Solid Edge part; units mm, degrees
sketch "Sketch1" plane through (0, 0, 0) normal (0, -1, 0) x (1, 0, 0)
  line L0 (-402.4784, 77.6999) -> (-342.4784, 77.6999)
  line L1 (-342.4784, 77.6999) -> (-342.4784, 477.6999)
  line L2 (-342.4784, 477.6999) -> (-402.4784, 477.6999)
  line L3 (-402.4784, 477.6999) -> (-402.4784, 77.6999)
  line L4 (-412.4784, 57.6999) -> (-332.4784, 57.6999)
  line L5 (-332.4784, 57.6999) -> (-332.4784, 587.6999)
  line L6 (-332.4784, 587.6999) -> (-412.4784, 587.6999)
  line L7 (-412.4784, 587.6999) -> (-412.4784, 57.6999)
  dimension "D1" = 402.4784
  dimension "D2" = 342.4784
  dimension "D3" = 332.4784
  dimension "D4" = 412.4784
extrude "Protrusion1" add sketch "Sketch1" against normal blind 50
sketch "Sketch2" plane through (-372.4784, 25, 77.6999) normal (0, 0, 1) x (1, 0, 0)
  circle A0 centre (0, 0) radius 10
extrude "Protrusion2" add sketch "Sketch2" along normal up to surface (400 mm away)
sketch "Sketch3" plane through (-372.4784, 50, 247.6999) normal (0, 1, 0) x (0, 0, 1)
  line L0 (290, -40) -> (340, -40)
  line L1 (340, -40) -> (340, 40)
  line L2 (340, 40) -> (290, 40)
  line L3 (290, 40) -> (290, -40)
  dimension "D1" = 290
  dimension "D2" = 340
extrude "ExtrudedProtrusion_3" add sketch "Sketch3" along normal blind 270
sketch "Sketch4" plane through (-372.4784, 310, 587.6999) normal (0, 0, 1) x (0, 1, 0)
  circle A0 centre (10, 0) radius 50
extrude "Cutout1" cut sketch "Sketch4" against normal through all
Design review of the part built by this model. Coordinates are the model's own, in mm. A direction names the side the tool comes from. Coordinates: 2 decimals unless noted, no trailing zeros. Order: outer loops, then holes, each group sorted by start corner. A loop starts at its lowest first (then second) coordinate and runs counter-clockwise, first axis right, second up. Notation, with made-up numbers: M -34.5,82.5 L -2.5,82.5 A32 ccw -2.5,112.5 Z; hole C -30,5.25 d5. An arc over 180 degrees is marked long. Answer as a JSON object with one key per item and string values. Group by question number.
1) Add section C-C, the plane x = -357.5. Write out the cut boundary in (y, z), then the cut area to 3 significant figures.
2) Tool access review of faces 1 (the flat face through (-372, 14, 477.7)), 2 (the flat face through (-342.478, 25, 275)), 3 (the flat face through (-340, 50, 334)): name each direction out of +Z, -Z, +X, -X, +Y, -Y from which nothing blocks a thin tool from reaching the whole face with its end or side.
3) Add section D-D, the plane y = 188.5. Write out the cut boundary in (x, z).
4) Wall thickness on L1, parallel to Z at x = -348, y = 122.5; L2, parallel to X at y = 32.5, z = 307; L3, parallel to Y at x = -403, z = 479: over which ranges is each line inside the solid? List them lowest first.
5) Add section B-B, the plane y = 25. Write out the cut boundary in (x, z).
6) Mouldability with a two-part tool opening along Z and no side actions: class faces 4 (the flat face through (-332.478, 48, 380)), 5 (the flat face through (-372, 168, 537.7)), 6 (the flat face through (-402.478, 25, 280)) as pulls with the +Z half, pulls with the -Z half, needs draft (parallel to the pull), parting line crosses it, or undercut.
7) Add section A-A, the plane z = 441. Write out the cut boundary in (x, y), then the cut area to 3 significant figures.
8) For pin 1 (1 mm diameter, centred on x = -402.5, y = 120.5, fed in from -Z); pin 2 (2 mm diameter, centred on x = -382, z = 513.5, fed in from +Y); pin 3 (24 mm diameter, centred on x = -371.5, z = 269, fed in from +Y), all flat-tipped, find the tip position at first contact; note any pin that passes through.
Computed values:
{
 "1": {"outline": "M 0,57.7 L 50,57.7 L 50,77.7 L 0,77.7 Z; M 0,477.7 L 50,477.7 L 50,537.7 L 272.3,537.7 L 272.3,587.7 L 0,587.7 Z", "area": "17,600 mm^2"},
 "2": {"face 1": "none", "face 2": "+Y, -Y", "face 3": "-Z, +X, -X, +Y"},
 "3": {"outline": "M -412.48,537.7 L -332.48,537.7 L -332.48,587.7 L -412.48,587.7 Z"},
 "4": {"L1": "z = 537.7 to 587.7", "L2": "x = -412.48 to -402.48, -379.09 to -365.86, -342.48 to -332.48", "L3": "y = 0 to 50"},
 "5": {"outline": "M -412.48,57.7 L -332.48,57.7 L -332.48,587.7 L -412.48,587.7 Z; hole M -402.48,77.7 L -382.48,77.7 L -382.48,477.7 L -402.48,477.7 Z; hole M -362.48,77.7 L -342.48,77.7 L -342.48,477.7 L -362.48,477.7 Z"},
 "6": {"face 4": "needs draft", "face 5": "pulls with the -Z half", "face 6": "undercut"},
 "7": {"outline": "M -412.48,0 L -402.48,0 L -402.48,50 L -412.48,50 Z; C -372.48,25 d20; M -342.48,0 L -332.48,0 L -332.48,50 L -342.48,50 Z", "area": "1,310 mm^2"},
 "8": {"pin 1": "stops at z = 537.7", "pin 2": "stops at y = 50", "pin 3": "stops at y = 35"}
}
